Geometry check sheet. Reference: the model listing, model coordinates, mm. Face numbers are marked on the shaded views. Round coordinates to 2 decimals unless told otherwise and drop trailing zeros. Write each loop counter-clockwise with the first axis right and the second up, starting at its lowest first coordinate (ties: lowest second). Pieces come first, ordered by that corner, then holes. Notation, with made-up numbers: M 35,-6.75 L 58,-6.75 A17 cw 58,26.25 Z; hole C 64,26.25 d5. An arc over 180 degrees is marked long. Use a Markdown table: item, result.
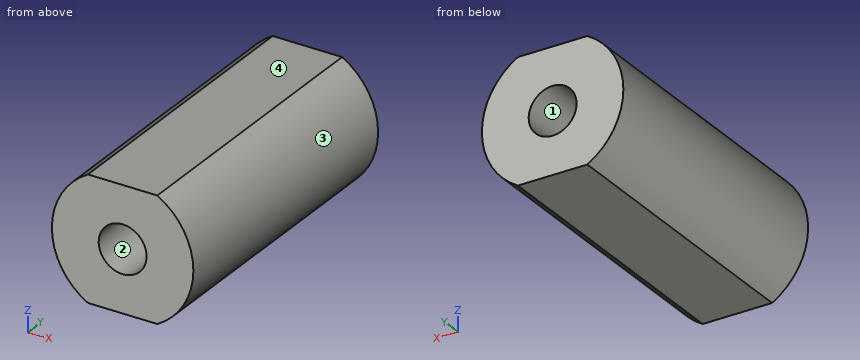
Autodesk Inventor part; units mm, degrees
ref_plane "YZ Plane" through (0, 0, 0) normal (1, 0, 0) x (0, 1, 0)
ref_plane "XZ Plane" through (0, 0, 0) normal (0, 1, 0) x (-1, 0, 0)
ref_plane "XY Plane" through (0, 0, 0) normal (0, 0, 1) x (1, 0, 0)
sketch "Sketch1" plane through (0, 0, 0) normal (0, 1, 0) x (-1, 0, 0)
  circle A0 centre (0, 0) radius 9.75
  line L0 (-9.75, -8.5) -> (9.75, -8.5)
  line L1 (9.75, -8.5) -> (9.75, 8.5)
  line L2 (9.75, 8.5) -> (-9.75, 8.5)
  line L3 (-9.75, 8.5) -> (-9.75, -8.5)
  line L4 (-9.75, -8.5) -> (9.75, 8.5) construction
  line L5 (9.75, -8.5) -> (-9.75, 8.5) construction
  point P0 (4.7762, 8.5)
  point P1 (-4.7762, 8.5)
  point P2 (-4.7762, -8.5)
  point P3 (4.7762, -8.5)
  dimension "d18" = 19.5
  dimension "d19" = 17
extrude "Extrusion1" add sketch "Sketch1" along normal mid plane 40 contours A0 L0 L2
sketch "Sketch2" plane through (0, 20, 0) normal (0, 1, 0) x (1, 0, 0)
  point P0 (0, 0)
hole "Hole1" at (0, 20, 0) direction (0, -1, 0) diameter 6.6 depth 10 tip angle 118
sketch "Sketch3" plane through (0, -20, 0) normal (0, -1, 0) x (1, 0, 0)
  point P0 (0, 0)
hole "Hole2" at (0, -20, 0) direction (0, 1, 0) diameter 6.6 depth 10 tip angle 118
properties part number "SP35V1 Vastago Cierre"
Item 1: Cross-section at C-C, the plane y = 6. Record the cut outline in (x, z).
Outcome:
| item | result |
|---|---|
| outline | M -4.78,-8.5 L 4.78,-8.5 A9.75 ccw 4.78,8.5 L -4.78,8.5 A9.75 ccw Z |
Item 2: Cross-section at B-B, the plane z = -3.75. Record the cut outline in (x, y), and give its area (3 significant figures).
Outcome:
| item | result |
|---|---|
| outline | M -9,-20 L 9,-20 L 9,20 L -9,20 Z |
| area | 720 mm2 |
Item 3: Cross-section at A-A, the plane y = -17. Record the cut outline in (x, z), and give its area (3 significant figures).
Outcome:
| item | result |
|---|---|
| outline | M -4.78,-8.5 L 4.78,-8.5 A9.75 ccw 4.78,8.5 L -4.78,8.5 A9.75 ccw Z; hole C 0,0 d6.6 |
| area | 248 mm2 |
Item 4: Material ranges on line 1 along Z through (x, y) = (0, 14.5); line 2 along X through (y, z) = (-13.5, 0); line 3 along Z through (x, y) = (2.75, 14), recorded low to high. Write a range as from..to.
Outcome:
| item | result |
|---|---|
| line 1 | z = -8.5..-3.3, 3.3..8.5 |
| line 2 | x = -9.75..-3.3, 3.3..9.75 |
| line 3 | z = -8.5..-1.82, 1.82..8.5 |
Item 5: Mould release check, pull along Z, two halves, no side actions. Record for the marked faces 1, 2, 3 and 4: +Z half, -Z half, draft (parallel to the pull), parting line (faces both ways), or undercut.
Outcome:
| item | result |
|---|---|
| face 1 | undercut |
| face 2 | undercut |
| face 3 | parting line |
| face 4 | +Z half |
Item 6: Go/stop test with flat-tipped pins: pin 1 (6 mm diameter, centred on y = 7, z = -4.5, fed in from -X); pin 2 (1 mm diameter, centred on y = -7.5, z = -2.5, fed in from -X). Record where each tip stops, or that it passes through.
Outcome:
| item | result |
|---|---|
| pin 1 | stops at x = -9.63 |
| pin 2 | stops at x = -9.54 |
